Read the model definition and answer for the solid it produces. Units are mm, in the model's axes. Face numbers are marked on the shaded views. A direction names the side the tool comes from. Give positions to 0.01 mm unless a question says otherwise; leave off trailing zeros. Order: outer loops, then holes, each group sorted by start corner. A loop starts at its lowest first (then second) coordinate and runs counter-clockwise, first axis right, second up.
```python
from build123d import *

# Parameters (mm, degrees)
SKETCH_1_W          = 10
SKETCH_1_H          = 6
SKETCH_1_R          = 2.5
EXTRUDE_1_DEPTH     = 6
SKETCH_2_W          = 10
SKETCH_2_H          = 9.6
SKETCH_2_R          = 2.5
EXTRUDE_2_DEPTH     = 5
CUT_EXTRUDE_1_DEPTH = 15


with BuildPart() as part:
    # 草图1 → 凸台-拉伸1 (new body)
    with BuildSketch(Plane.XY):
        Rectangle(SKETCH_1_W, SKETCH_1_H)
        Circle(SKETCH_1_R, mode=Mode.SUBTRACT)
    extrude(amount=EXTRUDE_1_DEPTH)

    # 草图2 → 凸台-拉伸2 (add)
    with BuildSketch(Plane.XY):
        Rectangle(SKETCH_2_W, SKETCH_2_H)
        Circle(SKETCH_2_R, mode=Mode.SUBTRACT)
    extrude(amount=EXTRUDE_2_DEPTH)

    # 草图3 → 切除-拉伸1 (cut)
    with BuildSketch(Plane(origin=(5, 0, 0), x_dir=(0, 0, -1), z_dir=(1, 0, 0))):
        with BuildLine():
            Line((0, 4.8), (-2.5, 4.8))
            ThreePointArc((-2.5, 4.8), (-0.662457295, 2.706011826), (0, 0))
            Line((0, 0), (0, 4.8))
        make_face()
        with BuildLine():
            Line((0, -4.8), (0, 0))
            ThreePointArc((0, 0), (-0.662457295, -2.706011826), (-2.5, -4.8))
            Line((-2.5, -4.8), (0, -4.8))
        make_face()
    extrude(amount=-CUT_EXTRUDE_1_DEPTH, mode=Mode.SUBTRACT)


solid = part.part
```
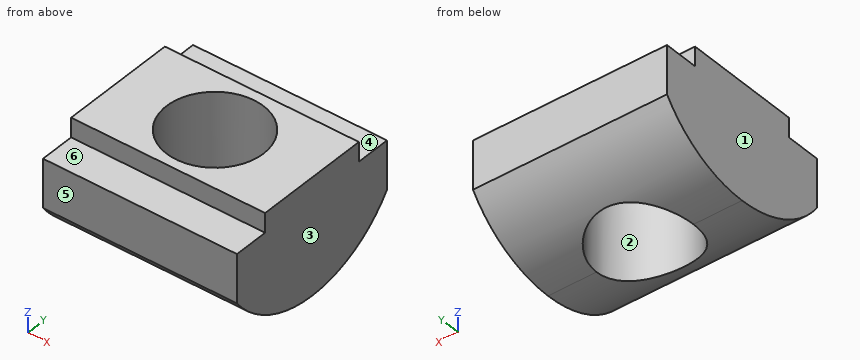
1) Consider L1, parallel to Y at x = 0, z = 3; L2, parallel to Y at x = 3.75, z = 5.25; L3, parallel to Y at x = 2, z = 1. Determine where each line is inside the solid, lowest interval first.
Final values:
L1: y = -4.8 to -2.5, 2.5 to 4.8
L2: y = -3 to 3
L3: y = -3.27 to -1.5, 1.5 to 3.27
2) The part is cut by section A-A on y = -1.5. Determine the outline of the cut face in (x, z), and give its area (3 significant figures).
Final values:
outline: (-5, 0.2) - (-2, 0.2) - (-2, 6) - (-5, 6) - close; (2, 0.2) - (5, 0.2) - (5, 6) - (2, 6) - close
area: 34.8 mm2
3) The part is cut by section B-B on x = -1.75. Determine the outline of the cut face in (y, z), and give its area (3 significant figures).
Final values:
outline: (-4.8, 2.5) arc R5.86 ccw to (-1.79, 0.28) - (-1.79, 6) - (-3, 6) - (-3, 5) - (-4.8, 5) - close; (1.79, 0.28) arc R5.86 ccw to (4.8, 2.5) - (4.8, 5) - (3, 5) - (3, 6) - (1.79, 6) - close
area: 25.7 mm2
4) For a pull along X with two mould halves and no side action, classify the marked faces 1, 2, 3 and 4 as released by +X, released by -X, zero draft, split by the parting line, or undercut.
Final values:
face 1: released by -X
face 2: undercut
face 3: released by +X
face 4: zero draft
5) Given pin 1 (3 mm diameter, centred on x = 0, y = 0, fed in from +Z); pin 2 (2 mm diameter, centred on x = 0.5, y = 2.5, fed in from -Z); pin 3 (4 mm diameter, centred on x = 3.5, y = 2.5, fed in from -Z); pin 4 (0.9 mm diameter, centred on x = 1, y = -3.5, fed in from +Z), each flat-ended and moving along its own axis, determine where each tip first touches the part or whether it passes through.
Final values:
pin 1: passes through
pin 2: stops at z = 0.38
pin 3: stops at z = 0.02
pin 4: stops at z = 5
6) A tool of negligible diameter and unlimited length cuts with its end or side. For the marked faces 5 and 6, from which of +Z, -Z, +X, -X, +Y, -Y can it reach the whole face along a straight path? Write none if from no direction.
Final values:
face 5: +Z, -Z, +X, -X, -Y
face 6: +Z, +X, -X, -Y
7) The part is cut by section D-D on y = 1. Determine the outline of the cut face in (x, z), and give its area (3 significant figures).
Final values:
outline: (-5, 0.09) - (-2.29, 0.09) - (-2.29, 6) - (-5, 6) - close; (2.29, 0.09) - (5, 0.09) - (5, 6) - (2.29, 6) - close
area: 32.0 mm2
8) The part is cut by section C-C on x = -3.75. Determine the outline of the cut face in (y, z).
Final values:
outline: (-4.8, 2.5) arc R5.86 ccw to (4.8, 2.5) - (4.8, 5) - (3, 5) - (3, 6) - (-3, 6) - (-3, 5) - (-4.8, 5) - close
